Source: CAD feature listing. Evaluate the final solid. Frame: model axes, mm. A direction names the side the tool comes from. Give positions to 0.01 mm unless a question says otherwise; leave off trailing zeros. Loops run counter-clockwise (first coordinate to the right, second up) from the corner with the lowest first, then second, coordinate; pieces in that order, holes last.
```python
from build123d import *

# Parameters (mm, degrees)
BOSS_EXTRUDE1_DEPTH = 38.1
BOSS_EXTRUDE3_DEPTH = 1


with BuildPart() as part:
    # Sketch1 → Boss-Extrude1 (new, symmetric)
    with BuildSketch(Plane(origin=(0, 0, 0), x_dir=(0, 0, -1), z_dir=(1, 0, 0))):
        Polygon((0, 0), (0, 42.1), (13.5, 42.1), (13.5, 0), (9.5, 0), (9.5, 38.1), (4, 38.1), (4, 0), align=None)
    extrude(amount=BOSS_EXTRUDE1_DEPTH, both=True)

    # Sketch2 → Boss-Extrude3 (add, symmetric)
    # profile 1 of 4: a face of its own
    with BuildSketch(Plane.XY):
        with BuildLine():
            Line((-22.865222246, 13.563040297), (-22.865222246, 18.780432709))
            Line((-22.865222246, 18.780432709), (-20.656196004, 18.780432709))
            add(Edge.make_bspline(
                [(-20.656196004, 18.780432709), (-20.41532138, 18.777714688), (-19.944746821, 18.772404742), (-19.256261279, 18.810224697), (-18.600645479, 18.877020485), (-17.978390446, 18.980226184), (-17.390247833, 19.12055906), (-16.836558282, 19.293424233), (-16.315862603, 19.49892128), (-15.828517725, 19.737297205), (-15.380553204, 20.022617586), (-14.993581031, 20.375797987), (-14.662017368, 20.786709496), (-14.391374272, 21.257071797), (-14.179098793, 21.785516775), (-14.024744286, 22.370402283), (-13.921962582, 23.01285099), (-13.903931965, 23.461547081), (-13.894568167, 23.694567371)],
                knots=[0, 0, 0, 0, 1.204916498, 2.353934341, 3.447552957, 4.50072552, 5.507144687, 6.470335232, 7.400410051, 8.305130608, 9.181490644, 10.047735884, 10.914032333, 11.813195112, 12.752367202, 13.754944245, 14.834080452, 16, 16, 16, 16], degree=3))
            add(Edge.make_bspline(
                [(-13.894568167, 23.694567371), (-13.903912104, 23.925417991), (-13.921898868, 24.369797661), (-14.025029441, 25.006807545), (-14.179399587, 25.587187383), (-14.389513591, 26.111548771), (-14.664177487, 26.574134139), (-14.993451519, 26.981011122), (-15.380818743, 27.330678309), (-15.828590089, 27.612940523), (-16.316667278, 27.84726287), (-16.836506867, 28.053338122), (-17.389829867, 28.226848133), (-17.978554423, 28.363192211), (-18.600944194, 28.462338902), (-19.256226176, 28.530250328), (-19.945228379, 28.567767567), (-20.416269188, 28.562489884), (-20.657613081, 28.559785795)],
                knots=[0, 0, 0, 0, 1.159335541, 2.231681874, 3.232698059, 4.170289135, 5.058653394, 5.923911943, 6.789704034, 7.666336687, 8.571988794, 9.505503644, 10.472256703, 11.481143997, 12.537323696, 13.634987235, 14.788254905, 16, 16, 16, 16], degree=3))
            Line((-20.657613081, 28.559785795), (-26.386965308, 28.563043481))
            Line((-26.386965308, 28.563043481), (-26.386965308, 13.563040297))
            Line((-26.386965308, 13.563040297), (-22.865222246, 13.563040297))
        make_face()
        with BuildLine():
            Line((-22.865222246, 25.667387508), (-20.544629022, 25.667387508))
            add(Edge.make_bspline(
                [(-20.544629022, 25.667387508), (-20.345180429, 25.665639397), (-19.962840192, 25.662288292), (-19.413885258, 25.59887468), (-18.918181922, 25.479214253), (-18.542791264, 25.333863497), (-18.279322093, 25.181576921), (-18.109546209, 25.041861769), (-17.964935401, 24.876369042), (-17.843038449, 24.687071269), (-17.752852301, 24.470987064), (-17.684339378, 24.233628804), (-17.637945851, 23.972355884), (-17.629418881, 23.789333614), (-17.625003742, 23.694567371)],
                knots=[0, 0, 0, 0, 1.781037572, 3.414224772, 4.923837313, 6.326680743, 6.992801752, 7.634335185, 8.281065082, 8.949094245, 9.636325156, 10.36458847, 11.153207937, 12, 12, 12, 12], degree=3))
            add(Edge.make_bspline(
                [(-17.625003742, 23.694567371), (-17.629329654, 23.597614693), (-17.637641958, 23.411318694), (-17.684922478, 23.144843592), (-17.752207557, 22.902812702), (-17.843064613, 22.682637579), (-17.964858791, 22.490072062), (-18.109429188, 22.321339009), (-18.279109983, 22.1782603), (-18.542470117, 22.021767063), (-18.917168662, 21.869595463), (-19.414049866, 21.749447311), (-19.962950296, 21.674835955), (-20.346487469, 21.675658964), (-20.546743492, 21.676088682)],
                knots=[0, 0, 0, 0, 0.858904102, 1.650396881, 2.391060107, 3.081381858, 3.751946835, 4.400513148, 5.042831016, 5.70833034, 7.106722173, 8.605996457, 10.227891054, 12, 12, 12, 12], degree=3))
            Line((-20.546743492, 21.676088682), (-22.865222246, 21.676088682))
            Line((-22.865222246, 21.676088682), (-22.865222246, 25.667387508))
        make_face(mode=Mode.SUBTRACT)
    # profile 2 of 4: a face of its own
    with BuildSketch(Plane.XY):
        Polygon((-12.195657947, 13.563043481), (-0.649855777, 13.563043481), (-0.649855777, 16.667391966), (-8.673914885, 16.667391966), (-8.673914885, 19.823911191), (-3.782845148, 19.823911191), (-3.782845148, 22.928262861), (-8.673914885, 22.928262861), (-8.673914885, 25.458691811), (-0.649855777, 25.458691811), (-0.649855777, 28.563043481), (-12.195657947, 28.563043481), align=None)
    # profile 3 of 4: a face of its own
    with BuildSketch(Plane.XY):
        Polygon((5.12608486, 25.458691811), (5.12608486, 13.563040297), (8.647827923, 13.563040297), (8.647827923, 25.458691811), (13.493818677, 25.458691811), (13.493818677, 28.563043481), (0.280094107, 28.563043481), (0.280094107, 25.458691811), align=None)
    # profile 4 of 4: a face of its own
    with BuildSketch(Plane.XY):
        with BuildLine():
            add(Edge.make_bspline(
                [(21.8608551, 13.354347785), (22.119813105, 13.358336117), (22.621956763, 13.366069866), (23.347309068, 13.45445267), (24.017283661, 13.603578733), (24.630497021, 13.811632782), (25.189445256, 14.078118279), (25.684655597, 14.415907315), (26.129733363, 14.807635649), (26.374895594, 15.114568002), (26.497831712, 15.268478626)],
                knots=[0, 0, 0, 0, 1.191138677, 2.309728683, 3.355722582, 4.344328933, 5.283888983, 6.195335572, 7.095054579, 8, 8, 8, 8], degree=3))
            Line((26.497831712, 15.268478626), (26.990503352, 13.563040297))
            Line((26.990503352, 13.563040297), (29.30869869, 13.563040297))
            Line((29.30869869, 13.563040297), (29.30869869, 22.088177976))
            Line((29.30869869, 22.088177976), (22.382852281, 22.088177976))
            Line((22.382852281, 22.088177976), (22.382852281, 19.203123016))
            Line((22.382852281, 19.203123016), (25.786955627, 19.203123016))
            Line((25.786955627, 19.203123016), (25.786955627, 18.774812166))
            add(Edge.make_bspline(
                [(25.786955627, 18.774812166), (25.778243203, 18.661219148), (25.761488992, 18.442776904), (25.702246402, 18.128562143), (25.614895527, 17.840434035), (25.497809633, 17.575930668), (25.346821564, 17.340790726), (25.16732423, 17.130707606), (24.957475692, 16.947308094), (24.63654282, 16.740507442), (24.194902065, 16.536753638), (23.629652259, 16.364249197), (23.028988663, 16.258629639), (22.6167514, 16.25292484), (22.405439539, 16.250000573)],
                knots=[0, 0, 0, 0, 0.861669082, 1.657011429, 2.414175731, 3.135788245, 3.838590194, 4.52112295, 5.220643916, 5.939296776, 7.403767205, 8.884228686, 10.402862886, 12, 12, 12, 12], degree=3))
            add(Edge.make_bspline(
                [(22.405439539, 16.250000573), (22.25960337, 16.255002366), (21.974358066, 16.26478552), (21.556473033, 16.323383598), (21.161578461, 16.4238954), (20.790499519, 16.565804834), (20.441850175, 16.742306557), (20.115717207, 16.958951958), (19.816347235, 17.219006913), (19.537082003, 17.513572772), (19.286190745, 17.845177479), (19.070603452, 18.215328788), (18.883726471, 18.617755475), (18.732087018, 19.05621736), (18.609948745, 19.528105564), (18.528810433, 20.035948609), (18.471242635, 20.57699171), (18.461518922, 20.949842028), (18.456525657, 21.141305959)],
                knots=[0, 0, 0, 0, 0.986869521, 1.930247473, 2.848904307, 3.738120068, 4.613047601, 5.488129678, 6.379987628, 7.290452962, 8.230384354, 9.186491415, 10.18353076, 11.227919754, 12.321393683, 13.477294155, 14.704554734, 16, 16, 16, 16], degree=3))
            add(Edge.make_bspline(
                [(18.456525657, 21.141305959), (18.462691715, 21.33059976), (18.47469819, 21.699190413), (18.534060968, 22.233041601), (18.62284679, 22.732163005), (18.751930806, 23.192563277), (18.905705346, 23.620561964), (19.100451259, 24.00895419), (19.321125945, 24.36633998), (19.58108987, 24.680617067), (19.860542252, 24.962795133), (20.162806955, 25.204508316), (20.481013939, 25.412390421), (20.817605993, 25.582469386), (21.172019795, 25.713956508), (21.544172891, 25.804526785), (21.934117354, 25.861522595), (22.200891059, 25.869009794), (22.336961264, 25.872828703)],
                knots=[0, 0, 0, 0, 1.319686362, 2.569677693, 3.740666748, 4.849050422, 5.89897666, 6.905298387, 7.872232364, 8.820039799, 9.741499591, 10.636028391, 11.512339942, 12.386520023, 13.259089862, 14.141114384, 15.051859528, 16, 16, 16, 16], degree=3))
            add(Edge.make_bspline(
                [(22.336961264, 25.872828703), (22.524294222, 25.867412582), (22.883466683, 25.857028283), (23.394731341, 25.772727742), (23.856558075, 25.649553589), (24.263315352, 25.470493213), (24.620629848, 25.258577476), (24.928723783, 25.018120229), (25.195978892, 24.759746675), (25.332326749, 24.561134201), (25.398918436, 24.464132752)],
                knots=[0, 0, 0, 0, 1.278335478, 2.450945646, 3.529594048, 4.533408079, 5.47533349, 6.35867971, 7.198386473, 8, 8, 8, 8], degree=3))
            Line((25.398918436, 24.464132752), (28.439218206, 25.700050346))
            add(Edge.make_bspline(
                [(28.439218206, 25.700050346), (28.361079034, 25.823929698), (28.206257037, 26.069379557), (27.948215698, 26.41541292), (27.668439938, 26.7372298), (27.369948167, 27.03715345), (27.048315584, 27.311527509), (26.708040547, 27.564420909), (26.345403709, 27.791997061), (25.963035389, 27.997909002), (25.564035608, 28.179099544), (25.150089409, 28.336749678), (24.722958781, 28.469607783), (24.281431216, 28.581812576), (23.825986668, 28.665722756), (23.3566313, 28.723737703), (22.874502715, 28.760511724), (22.547897044, 28.765803507), (22.382613447, 28.768481492)],
                knots=[0, 0, 0, 0, 0.987447504, 1.956491095, 2.907400243, 3.861102247, 4.807224743, 5.755757746, 6.717677965, 7.691726565, 8.682375344, 9.670716339, 10.676890986, 11.697355627, 12.741116498, 13.797592121, 14.885439147, 16, 16, 16, 16], degree=3))
            add(Edge.make_bspline(
                [(22.382613447, 28.768481492), (22.099730981, 28.758621488), (21.546339814, 28.739332773), (20.738378686, 28.639019262), (19.976200826, 28.471654692), (19.256240644, 28.248028091), (18.582018051, 27.956846547), (17.953235542, 27.602814057), (17.366836258, 27.189513377), (16.831285034, 26.712718675), (16.342994106, 26.186120845), (15.920267276, 25.60388094), (15.560854464, 24.974654528), (15.262488717, 24.299715759), (15.031227955, 23.576774675), (14.863080191, 22.807064787), (14.753855008, 21.989948886), (14.733332745, 21.428607179), (14.722829213, 21.141305959)],
                knots=[0, 0, 0, 0, 1.115331854, 2.181877176, 3.203772788, 4.187522244, 5.148954065, 6.092764476, 7.027114261, 7.971051081, 8.914054022, 9.852422535, 10.800463299, 11.765325617, 12.755760334, 13.786945325, 14.86733286, 16, 16, 16, 16], degree=3))
            add(Edge.make_bspline(
                [(14.722829213, 21.141305959), (14.730391549, 20.847575412), (14.745163979, 20.273795857), (14.84038858, 19.438408616), (14.994067089, 18.651412225), (15.200032703, 17.912316957), (15.469382319, 17.22226235), (15.794902903, 16.581399506), (16.179745575, 15.988990666), (16.61978942, 15.447409763), (17.111798353, 14.960441635), (17.653299929, 14.536564006), (18.241912503, 14.179583732), (18.876009186, 13.884113096), (19.55662642, 13.654005492), (20.282457402, 13.483895793), (21.054564416, 13.378322793), (21.585535664, 13.362470658), (21.857613336, 13.354347785)],
                knots=[0, 0, 0, 0, 1.181046208, 2.307081006, 3.375954413, 4.402557026, 5.387877309, 6.349572523, 7.287872367, 8.223031757, 9.150200772, 10.065592574, 10.981568491, 11.912305234, 12.87289741, 13.865182061, 14.906087104, 16, 16, 16, 16], degree=3))
            Line((21.857613336, 13.354347785), (21.8608551, 13.354347785))
        make_face()
    extrude(amount=BOSS_EXTRUDE3_DEPTH, both=True)


solid = part.part
```
(1) Section B-B, the plane x = 2. Return the cut outline in (y, z).
A:
outline: (0, -13.5) - (42.1, -13.5) - (42.1, 0) - (28.56, 0) - (28.56, 1) - (25.46, 1) - (25.46, 0) - (0, 0) - (0, -4) - (38.1, -4) - (38.1, -9.5) - (0, -9.5) - close
(2) First-contact query: pin 1 (0.5 mm diameter, centred on y = 23, z = 0.5, fed in from -X); pin 2 (0.8 mm diameter, centred on x = 10, z = 0.5, fed in from +Y); pin 3 (0.5 mm diameter, centred on y = 15.5, z = 0.5, fed in from +X). Flat tips, straight axial feed; report the tip coordinate or a pass-through.
A:
pin 1: stops at x = -26.39
pin 2: stops at y = 28.56
pin 3: stops at x = 29.31
(3) Section C-C, the plane z = -5. Return the cut outline in (x, y).
A:
outline: (-38.1, 38.1) - (38.1, 38.1) - (38.1, 42.1) - (-38.1, 42.1) - close
(4) Section A-A, the plane y = 35. Return the cut outline in (x, z).
A:
outline: (-38.1, -13.5) - (38.1, -13.5) - (38.1, -9.5) - (-38.1, -9.5) - close; (-38.1, -4) - (38.1, -4) - (38.1, 0) - (-38.1, 0) - close
(5) Ray query, line 1 along Z through (x, y) = (19, 29); line 2 along Z through (x, y) = (-2, 25.5); line 3 along X through (y, z) = (23.5, 0.5). Return the intervals inside material, ascending.
A:
line 1: z = -13.5 to -9.5, -4 to 0
line 2: z = -13.5 to -9.5, -4 to 1
line 3: x = -26.39 to -22.87, -17.64 to -13.9, -12.2 to -8.67, 5.13 to 8.65, 15.02 to 18.87
(6) Mould query, pull axis Z, two halves, no side actions, for faces 1 (the flat face through (1, 0, -2)), 2 (the flat face through (1, 21, -13.5)), 3 (the flat face through (1, 19, -9.5)). Classes: pulls with the +Z half, pulls with the -Z half, needs draft (parallel to the pull), parting line crosses it, or undercut.
A:
face 1: needs draft
face 2: pulls with the -Z half
face 3: undercut
(7) Section D-D, the plane x = -25.5. Return the cut outline in (y, z).
A:
outline: (0, -13.5) - (42.1, -13.5) - (42.1, 0) - (28.56, 0) - (28.56, 1) - (13.56, 1) - (13.56, 0) - (0, 0) - (0, -4) - (38.1, -4) - (38.1, -9.5) - (0, -9.5) - close
(8) Reachability of faces 4 (the flat face through (-22, 21, 1)), 5 (the flat face through (-20, 24, 0)), 6 (the flat face through (1, 19, -4)) from +Z, -Z, +X, -X, +Y, -Y: full face, straight path, thin tool, end or side. Return the list, or none.
A:
face 4: +Z, +X, -X, +Y, -Y
face 5: +Z
face 6: +X, -X, -Y
